from build123d import *

# Parameters (mm, degrees)
F1_DEPTH = 42
F2_R     = 10
F3_DEPTH = 55
F4_R     = 1.5
F5_DEPTH = 197.5


with BuildPart() as f1:
    # F0 (on Front) → F1 (new body)
    with BuildSketch(Plane.XZ):
        Polygon((-127.40964, 0), (172.59036, 0), (172.59036, 70), (-127.40964, 20), align=None)
    extrude(amount=-F1_DEPTH)

    # F2 (on face) → F3 (cut)
    with BuildSketch(Plane.YZ.offset(172.59036)):
        with Locations((21, 35)):
            Circle(F2_R)
    extrude(amount=-F3_DEPTH, mode=Mode.SUBTRACT)

    # F4 (on face) → F5 (cut)
    with BuildSketch(Plane.XZ):
        with Locations((-115.736268, 5.088853)):
            Circle(F4_R)
        with Locations((148.481086, 5.088853)):
            Circle(F4_R)
    extrude(amount=-F5_DEPTH, mode=Mode.SUBTRACT)


solid = f1.part
Geometry check sheet. Reference: the model listing, model coordinates, mm. A direction names the side the tool comes from. Coordinates: 2 decimals unless noted, no trailing zeros. Write each loop counter-clockwise with the first axis right and the second up, starting at its lowest first coordinate (ties: lowest second). Pieces come first, ordered by that corner, then holes. Notation, with made-up numbers: (41, 37) -> (67, 37) arc R9 ccw to (67, 45) -> close; hole circle Ø1 at (3.5, -6). An arc over 180 degrees is marked (long way). One line per question, with ' | ' between items.
1. Cross-section at C-C on z = 35. Record the cut outline in (x, y), and give its area (3 significant figures).
Answers:
outline: (-37.41, 0) -> (172.59, 0) -> (172.59, 11) -> (117.59, 11) -> (117.59, 31) -> (172.59, 31) -> (172.59, 42) -> (-37.41, 42) -> close | area: 7,720 mm²
2. Draft check along Z on faces 1 (the flat face through (172.59, 11, 27)), 2 (the flat face through (20, 21, 0)), 3 (the flat face through (24.69, 20.71, 45.35)), 4 (the flat face through (117.59, 21, 35)). Enter one of: +Z half, -Z half, draft (parallel to the pull), parting line (faces both ways), or undercut.
Answers:
face 1: draft | face 2: -Z half | face 3: +Z half | face 4: undercut
3. Depth check by flat-ended pin: pin 1 Ø1.5 at (x, y) = (31, 8.5) entering from +Z; pin 2 Ø4 at (x, z) = (112.5, 37) entering from -Y; pin 3 Ø2 at (x, y) = (-97, 26.5) entering from +Z; pin 4 Ø8 at (x, y) = (58, 35) entering from +Z. Enter the tip coordinate at first touch or a pass-through.
Answers:
pin 1: stops at z = 46.53 | pin 2: stops at y = 0 | pin 3: stops at z = 25.23 | pin 4: stops at z = 51.57
4. Cross-section at D-D on y = 37. Record the cut outline in (x, z), and give its area (3 significant figures).
Answers:
outline: (-127.41, 0) -> (172.59, 0) -> (172.59, 70) -> (-127.41, 20) -> close; hole circle Ø3 at (-115.74, 5.09); hole circle Ø3 at (148.48, 5.09) | area: 13,500 mm²
5. Cross-section at A-A on y = 14.5. Record the cut outline in (x, z).
Answers:
outline: (-127.41, 0) -> (172.59, 0) -> (172.59, 27.4) -> (117.59, 27.4) -> (117.59, 42.6) -> (172.59, 42.6) -> (172.59, 70) -> (-127.41, 20) -> close; hole circle Ø3 at (-115.74, 5.09); hole circle Ø3 at (148.48, 5.09)
6. Cross-section at B-B on x = 121. Record the cut outline in (y, z), and give its area (3 significant figures).
Answers:
outline: (0, 0) -> (42, 0) -> (42, 61.4) -> (0, 61.4) -> close; hole circle Ø20 at (21, 35) | area: 2,260 mm²
7. Set-up check for faces 5 (the cylindrical face through (145.475, 25.614, 26.128)), 6 (the flat face through (-127.41, 21, 10)): record each of +Z, -Z, +X, -X, +Y, -Y from which the full face is reachable in a straight line by a thin tool's end or side.
Answers:
face 5: +X | face 6: +Z, -Z, -X, +Y, -Y
8. Thickness scan on probe 1 along Z at (x, y) = (134, 28); probe 2 along Z at (x, y) = (122.5, 20); probe 3 along Z at (x, y) = (-89, 32). Record the ranges inside material, lowest first. Write a range as from..to.
Answers:
probe 1: z = 0..27.86, 42.14..63.57 | probe 2: z = 0..25.05, 44.95..61.65 | probe 3: z = 0..26.4
